Verification items for this drawing (mm, ordinates from the low corner). A direction names the side the tool comes from. Round coordinates to 2 decimals unless told otherwise and drop trailing zeros. Order: outer loops, then holes, each group sorted by start corner. A loop starts at its lowest first (then second) coordinate and runs counter-clockwise, first axis right, second up. Notation, with made-up numbers: (35, 27) - (90, 27) arc R18 ccw to (90, 39) - close; hole circle Ø8 at (-6.75, 81). An arc over 180 degrees is marked (long way). Use a Markdown table: item, result. Add a question column.
(1) Section check A-A on y = 48. Record the boundary of the cut face in (x, z), then the cut area to 3 significant figures.
(2) Section check C-C on z = 56.5. Record the boundary of the cut face in (x, y), then the cut area to 3 significant figures.
(3) Access from +Z, -Z, +X, -X, +Y, -Y to the whole of each face (thin tool, end or side, straight path). Record for the marked faces 4 and 5.
(4) Mould release check, pull along Z, two halves, no side actions. Record for the marked faces 1, 2 and 3: released by +Z, released by -Z, zero draft, split by the parting line, or undercut.
(5) Section check B-B on x = 25. Record the boundary of the cut face in (y, z).
(6) Gauge pin test, flat ends, axial feed: P1, Ø1, axis at y = 78.5, z = 2, coming from the +X side; P2, Ø1.8, axis at y = 78.5, z = 61, coming from the -X side; P3, Ø6, axis at x = 22, z = 10.5, coming from the +Y side. Record the tip position at first contact, or that the pin passes through.
(7) Thickness scan on line 1 along Z through (x, y) = (12.5, 43); line 2 along Y through (x, z) = (35.5, 54); line 3 along X through (y, z) = (23, 3.5). Record the ranges inside material, lowest first. Write a range as [from, to].
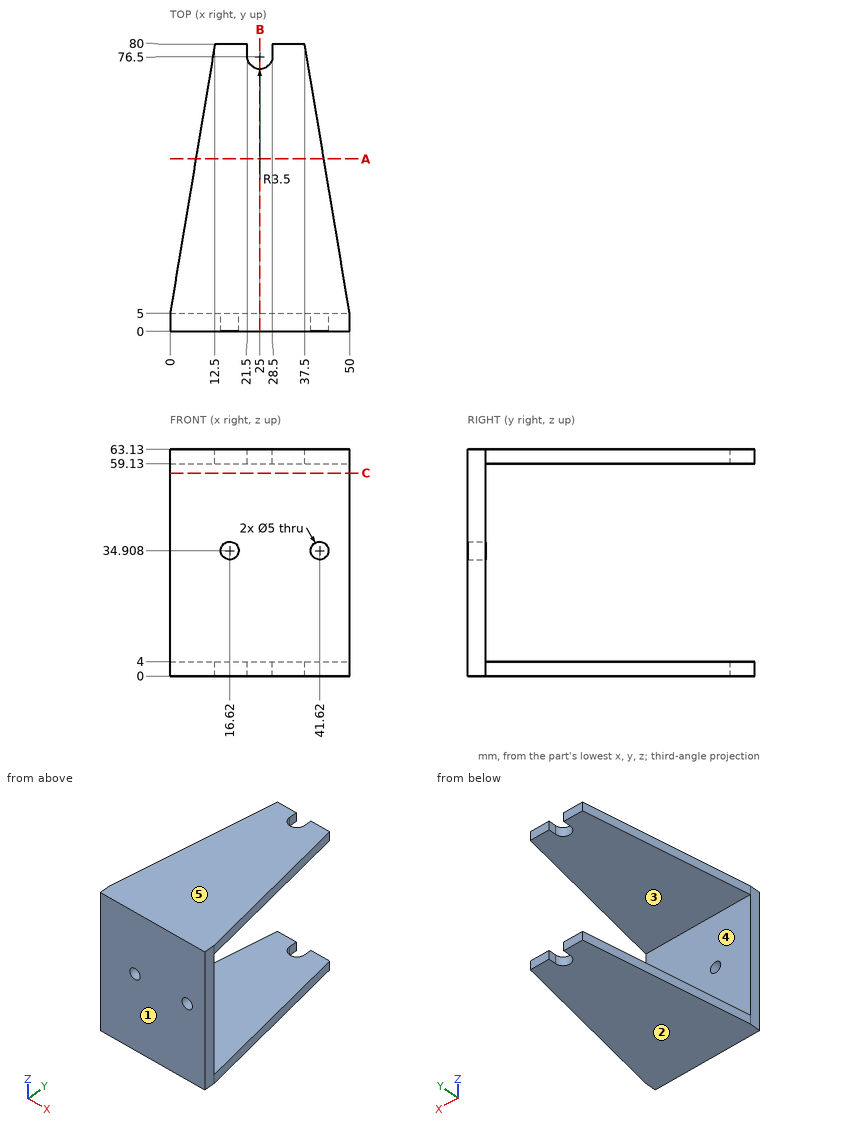
Check sheet entries:
| question | item | result |
|---|---|---|
| 1 | outline | (7.17, 0) - (42.83, 0) - (42.83, 4) - (7.17, 4) - close; (7.17, 59.13) - (42.83, 59.13) - (42.83, 63.13) - (7.17, 63.13) - close |
| 1 | area | 285 mm2 |
| 2 | outline | (0, 0) - (50, 0) - (50, 5) - (0, 5) - close |
| 2 | area | 250 mm2 |
| 3 | face 4 | +X, -X, +Y |
| 3 | face 5 | +Z, +X, -X, +Y, -Y |
| 4 | face 1 | zero draft |
| 4 | face 2 | released by -Z |
| 4 | face 3 | undercut |
| 5 | outline | (0, 0) - (73, 0) - (73, 4) - (5, 4) - (5, 59.13) - (73, 59.13) - (73, 63.13) - (0, 63.13) - close |
| 6 | P1 | stops at x = 37.83 |
| 6 | P2 | stops at x = 12.1 |
| 6 | P3 | stops at y = 5 |
| 7 | line 1 | z = [0, 4], [59.13, 63.13] |
| 7 | line 2 | y = [0, 5] |
| 7 | line 3 | x = [3, 47] |
